Job drawing, mm, ordinate dimensions from the low corner. One solid piece. Coordinates: 2 decimals unless noted, no trailing zeros. Write each loop counter-clockwise with the first axis right and the second up, starting at its lowest first coordinate (ties: lowest second). Pieces come first, ordered by that corner, then holes.
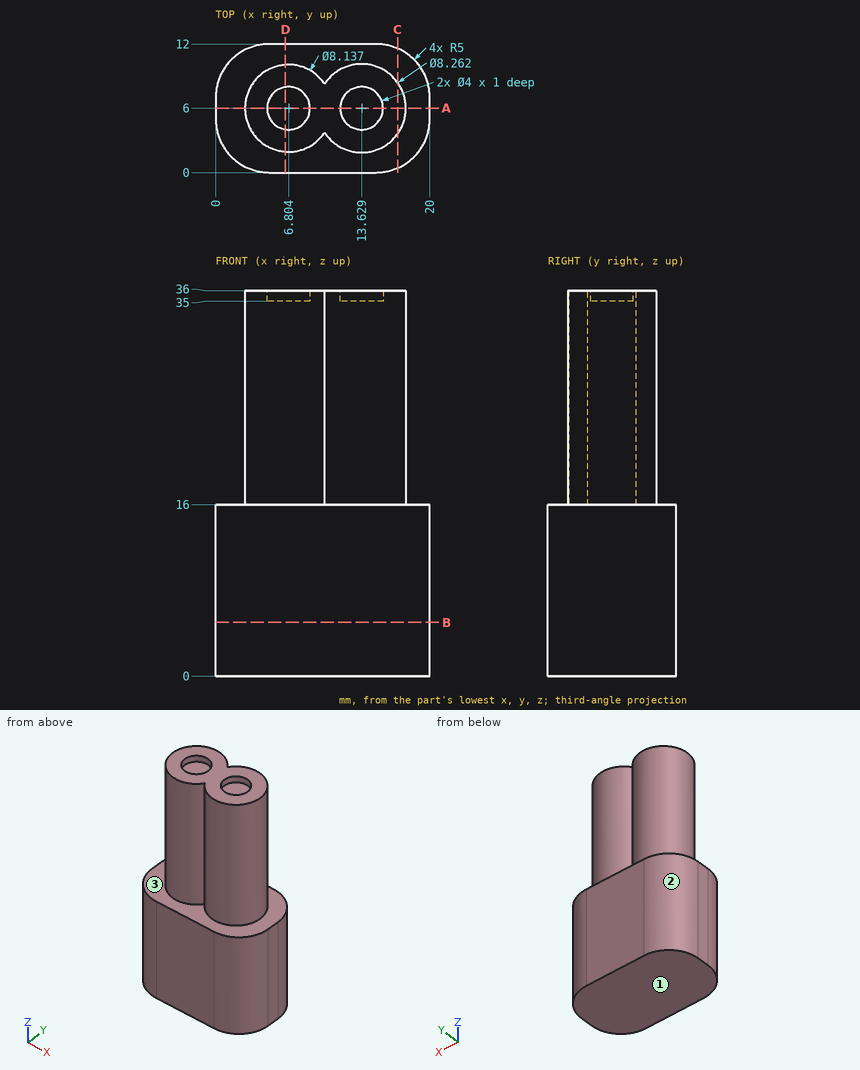
1. Mould opens along Z. For the marked faces 1, 2 and 3 say: +Z half, -Z half, draft (parallel to the pull), parting line (faces both ways), or undercut.
Computed values:
face 1: -Z half
face 2: draft
face 3: +Z half
2. Saw through at A-A on y = 6. List the corners of the cut face in (x, z) (1 decimal).
Computed values:
outline: (0, 0) - (20, 0) - (20, 16) - (17.8, 16) - (17.8, 36) - (15.6, 36) - (15.6, 35) - (11.6, 35) - (11.6, 36) - (8.8, 36) - (8.8, 35) - (4.8, 35) - (4.8, 36) - (2.7, 36) - (2.7, 16) - (0, 16) - close
3. Saw through at C-C on x = 17. List the corners of the cut face in (y, z), plus the area to 3 significant figures.
Computed values:
outline: (0.42, 0) - (11.58, 0) - (11.58, 16) - (8.39, 16) - (8.39, 36) - (3.61, 36) - (3.61, 16) - (0.42, 16) - close
area: 274 mm2
4. Flat gauge pins, fed straight in: pin 1 (4 mm diameter, centred on x = 16, z = 30.5, fed in from -Y) (1 decimal); pin 2 (10 mm diameter, centred on x = 5, z = 32, fed in from +Y). Where does each tip first touch, or does it go through?
Computed values:
pin 1: stops at y = 1.9
pin 2: stops at y = 10.07
5. Saw through at D-D on x = 6.5. List the corners of the cut face in (y, z), plus the area to 3 significant figures.
Computed values:
outline: (0, 0) - (12, 0) - (12, 16) - (10.06, 16) - (10.06, 36) - (7.98, 36) - (7.98, 35) - (4.02, 35) - (4.02, 36) - (1.94, 36) - (1.94, 16) - (0, 16) - close
area: 350 mm2
6. Saw through at B-B on z = 5. List the corners of the cut face in (x, y).
Computed values:
outline: (0, 5) arc R5 ccw to (5, 0) - (15, 0) arc R5 ccw to (20, 5) - (20, 7) arc R5 ccw to (15, 12) - (5, 12) arc R5 ccw to (0, 7) - close
7. Probe line 1 along Z through (x, y) = (12, 5.5); line 2 along Z through (x, y) = (15.75, 10.75); line 3 along X through (y, z) = (7.25, 6.5). List the from-to ranges inside material, lowest first.
Computed values:
line 1: z = 0 to 35
line 2: z = 0 to 16
line 3: x = 0.01 to 19.99
